Geometry check sheet. Reference: the model listing, model coordinates, mm. A direction names the side the tool comes from. Coordinates: 2 decimals unless noted, no trailing zeros. Loops run counter-clockwise (first coordinate to the right, second up) from the corner with the lowest first, then second, coordinate; pieces in that order, holes last. Notation, with made-up numbers: (11, 86) - (24, 86) arc R20 ccw to (24, 121) - close; hole circle Ø3 at (11, 87.5). An arc over 180 degrees is marked (long way). Write each question's results on one line, items separated by ' | '. Start each with the question number.
(1) Sectioned sample at C-C (x = 3.5). Enter the section's corners in (y, z).
(2) Sectioned sample at B-B (z = -4). Enter the section's corners in (x, y).
(3) Sectioned sample at A-A (x = 17). Enter the section's corners in (y, z).
(4) Sectioned sample at D-D (z = -30.5). State how many separate pieces and enclosed holes the cut face has, plus the area to 3 significant figures.
(5) Material ranges on probe 1 along Y at (x, z) = (36, -10); probe 2 along Z at (x, y) = (3.5, 47.1); probe 3 along Y at (x, z) = (15, -9), recorded low to high.
(6) Go/stop test with flat-tipped pins: pin 1 Ø4 at (x, z) = (30.5, -31) entering from -Y; pin 2 Ø3 at (y, z) = (36, -13.5) entering from -X. Record where each tip stops, or that it passes through.
(7) Access from +Z, -Z, +X, -X, +Y, -Y to the whole of each face (thin tool, end or side, straight path). Record for faces 1 (the face through (16, 5, -19)), 2 (the face through (28.914, 46.965, -4.208)).
(8) Mould release check, pull along Y, two halves, no side actions. Record for faces 3 (the face through (17, 44.5, -19)), 4 (the face through (19, 49.5, -18)), 5 (the face through (0, 2, -24)), 6 (the face through (33, 24, -24)): pulls with the +Y half, pulls with the -Y half, needs draft (parallel to the pull), parting line crosses it, or undercut.
Autodesk Inventor part; units mm, degrees
ref_plane "YZ Plane" through (0, 0, 0) normal (1, 0, 0) x (0, 1, 0)
ref_plane "XZ Plane" through (0, 0, 0) normal (0, 1, 0) x (-1, 0, 0)
ref_plane "XY Plane" through (0, 0, 0) normal (0, 0, 1) x (1, 0, 0)
sketch "スケッチ1" plane through (0, 0, 0) normal (0, 1, 0) x (-1, 0, 0)
  line L0 (0, 0) -> (-38, 0)
  line L1 (-38, 0) -> (-38, -48)
  line L2 (-38, -48) -> (0, -48)
  line L3 (0, -48) -> (0, 0)
  dimension "d0" = 48
  dimension "d1" = 38
extrude "押し出し1" add sketch "スケッチ1" along normal blind 49.5
sketch "スケッチ2" plane through (38, 0, -48) normal (0, 0, -1) x (-1, 0, 0)
  line L0 (5, 44.5) -> (59.072, 44.5)
  line L1 (59.072, 44.5) -> (59.072, 5)
  line L2 (59.072, 5) -> (5, 5)
  line L3 (5, 5) -> (5, 44.5)
  line L4 (0, 49.5) -> (38, 49.5)
  line L5 (0, 0) -> (38, 0)
  line L6 (0, 0) -> (0, 49.5)
  dimension "d4" = 39.5
  dimension "d6" = 5
  dimension "d7" = 5
extrude "押し出し2" cut sketch "スケッチ2" against normal blind 100
sketch "スケッチ3" plane through (0, 49.5, 0) normal (0, 1, 0) x (1, 0, 0)
  line L0 (38, 48) -> (0, 48)
  line L1 (38, 0) -> (38, 48)
  point P0 (0, 0)
  point P1 (17, 32)
  dimension "d10" = 16
  dimension "d11" = 21
hole "穴1" at (17, 49.5, -32) direction (0, -1, 0) diameter 22 end through all
sketch "スケッチ4" plane through (0, 49.5, 0) normal (0, 1, 0) x (1, 0, 0)
  line L0 (0, 0) -> (38, 0)
  line L1 (38, 0) -> (38, 48)
  point P0 (30.5, 4)
  point P1 (30.5, 31)
  point P2 (3.5, 4)
  point P3 (3.5, 31)
  point P4 (3.5, 4)
  dimension "d19" = 4
  dimension "d20" = 7.5
  dimension "d23" = 27
  dimension "d26" = 27
hole "穴2" at (30.5, 49.5, -4) at (30.5, 49.5, -31) at (3.5, 49.5, -31) at (3.5, 49.5, -4) direction (0, -1, 0) diameter 3.2 end through all
sketch "スケッチ6" plane through (38, 0, 0) normal (1, 0, 0) x (0, 0, -1)
  line L0 (0, 49.5) -> (48, 49.5)
  line L1 (0, 0) -> (0, 49.5)
  point P0 (10, 34.5)
  point P1 (32, 34.5)
  point P2 (10, 19.5)
  point P3 (32, 19.5)
  dimension "d45" = 15
  dimension "d46" = 10
  dimension "d49" = 22
  dimension "d52" = 15
hole "穴4" at (38, 34.5, -10) at (38, 34.5, -32) at (38, 19.5, -10) at (38, 19.5, -32) direction (-1, 0, 0) diameter 1 end through all
properties part number "サーボモータ固定２軸"
Outcome:
1) outline: (0, -48) - (5, -48) - (5, -32.6) - (0, -32.6) - close; (0, -29.4) - (5, -29.4) - (5, -5.6) - (0, -5.6) - close; (0, -2.4) - (5, -2.4) - (5, 0) - (0, 0) - close; (44.5, -48) - (49.5, -48) - (49.5, -32.6) - (44.5, -32.6) - close; (44.5, -29.4) - (49.5, -29.4) - (49.5, -5.6) - (44.5, -5.6) - close; (44.5, -2.4) - (49.5, -2.4) - (49.5, 0) - (44.5, 0) - close
2) outline: (0, 0) - (1.9, 0) - (1.9, 5) - (0, 5) - close; (0, 44.5) - (1.9, 44.5) - (1.9, 49.5) - (0, 49.5) - close; (5.1, 0) - (28.9, 0) - (28.9, 5) - (5.1, 5) - close; (5.1, 44.5) - (28.9, 44.5) - (28.9, 49.5) - (5.1, 49.5) - close; (32.1, 0) - (38, 0) - (38, 49.5) - (32.1, 49.5) - (32.1, 44.5) - (33, 44.5) - (33, 5) - (32.1, 5) - close
3) outline: (0, -48) - (5, -48) - (5, -43) - (0, -43) - close; (0, -21) - (5, -21) - (5, 0) - (0, 0) - close; (44.5, -48) - (49.5, -48) - (49.5, -43) - (44.5, -43) - close; (44.5, -21) - (49.5, -21) - (49.5, 0) - (44.5, 0) - close
4) separate pieces: 7 | enclosed holes: 0 | area: 299 mm2
5) probe 1: y = 0 to 19, 20 to 34, 35 to 49.5 | probe 2: z = -48 to -32.6, -29.4 to -5.6, -2.4 to 0 | probe 3: y = 0 to 5, 44.5 to 49.5
6) pin 1: stops at y = 0 | pin 2: stops at x = 33
7) face 1: +Z, -Z, -X | face 2: +Y, -Y
8) face 3: undercut | face 4: pulls with the +Y half | face 5: needs draft | face 6: undercut
